CAD build for the part. Positions are in the model's coordinates, mm. A direction names the side the tool comes from. Coordinates: 2 decimals unless noted, no trailing zeros. Loops run counter-clockwise (first coordinate to the right, second up) from the corner with the lowest first, then second, coordinate; pieces in that order, holes last. Notation, with made-up numbers: (8, -19) -> (31, -19) arc R27 ccw to (31, 14) -> close; hole circle Ø4 at (-24.5, 32.25). An arc over 180 degrees is marked (long way). Write each question's results on one line, items separated by ' | '.
from build123d import *

# Parameters (mm, degrees)
SKETCH1_R               = 42.75
SKETCH1_R_2             = 38.75
BOSS_EXTRUDE1_DEPTH     = 20
BOSS_EXTRUDE2_DEPTH     = 15
SKETCH3_R               = 1.75
CUT_EXTRUDE1_DEPTH      = 43.75
CUT_EXTRUDE1_DEPTH_BACK = 43.75
SKETCH4_R               = 1.75
CUT_EXTRUDE2_DEPTH      = 43.7500001
CUT_EXTRUDE2_DEPTH_BACK = 43.7500001
FILLET1_R               = 2


with BuildPart() as part:
    # Sketch1 → Boss-Extrude1 (new body)
    with BuildSketch(Plane(origin=(0, 0, 0), x_dir=(1, 0, 0), z_dir=(0, 1, 0))):
        Circle(SKETCH1_R)
        Circle(SKETCH1_R_2, mode=Mode.SUBTRACT)
    extrude(amount=BOSS_EXTRUDE1_DEPTH)

    # Sketch2 → Boss-Extrude2 (add)
    with BuildSketch(Plane.XZ):
        with BuildLine():
            Line((40.171859539, 14.621361127), (36.413089055, 13.253280554))
            ThreePointArc((36.413089055, 13.253280554), (38.161300429, 6.728866885), (38.75, 0))
            Line((38.75, 0), (42.75, 0))
            ThreePointArc((42.75, 0), (42.100531441, 7.423459595), (40.171859539, 14.621361127))
        make_face()
        with BuildLine():
            Line((-7.423459595, -42.100531441), (-6.728866885, -38.161300429))
            ThreePointArc((-6.728866885, -38.161300429), (-13.253280554, -36.413089056), (-19.375, -33.558484397))
            Line((-19.375, -33.558484397), (-21.375, -37.022586012))
            ThreePointArc((-21.375, -37.022586012), (-14.621361127, -40.171859539), (-7.423459595, -42.100531441))
        make_face()
        with BuildLine():
            Line((-32.748399943, 27.479170314), (-29.684222171, 24.908019875))
            ThreePointArc((-29.684222171, 24.908019875), (-24.908019875, 29.684222171), (-19.375, 33.558484397))
            Line((-19.375, 33.558484397), (-21.375, 37.022586012))
            ThreePointArc((-21.375, 37.022586012), (-27.479170314, 32.748399943), (-32.748399943, 27.479170314))
        make_face()
    extrude(amount=BOSS_EXTRUDE2_DEPTH)

    # Sketch3 → Cut-Extrude1 (cut, two sides)
    with BuildSketch(Plane.XY) as cut_extrude1_sk:
        with Locations((0, 10)):
            Circle(SKETCH3_R)
    extrude(amount=CUT_EXTRUDE1_DEPTH, mode=Mode.SUBTRACT)
    extrude(cut_extrude1_sk.sketch, amount=-CUT_EXTRUDE1_DEPTH_BACK, mode=Mode.SUBTRACT)

    # Sketch4 → Cut-Extrude2 (cut, two sides)
    with BuildSketch(Plane(origin=(0, 0, 0), x_dir=(0, 0, -1), z_dir=(1, 0, 0))) as cut_extrude2_sk:
        with Locations((0, 10)):
            Circle(SKETCH4_R)
    extrude(amount=CUT_EXTRUDE2_DEPTH, mode=Mode.SUBTRACT)
    extrude(cut_extrude2_sk.sketch, amount=-CUT_EXTRUDE2_DEPTH_BACK, mode=Mode.SUBTRACT)

    # Fillet1
    fillet1_edges = [part.edges().sort_by_distance(p)[0] for p in [
        (-42.75, 20, 0),
    ]]
    fillet(fillet1_edges, radius=FILLET1_R)


solid = part.part
1) Slice it at C-C (y = 10). Write the cut outline in (x, z), then the cut area to 3 significant figures.
Outcome:
outline: (-42.71, -1.75) arc R42.75 ccw to (-1.75, -42.71) -> (-1.75, -38.71) arc R38.75 cw to (-38.71, -1.75) -> close; (-42.71, 1.75) -> (-38.71, 1.75) arc R38.75 cw to (-1.75, 38.71) -> (-1.75, 42.71) arc R42.75 ccw to start; (1.75, -42.71) arc R42.75 ccw to (42.71, -1.75) -> (38.71, -1.75) arc R38.75 cw to (1.75, -38.71) -> close; (1.75, 38.71) arc R38.75 cw to (38.71, 1.75) -> (42.71, 1.75) arc R42.75 ccw to (1.75, 42.71) -> close | area: 968 mm^2
2) Pin check, flat tips, straight feed: pin 1 (21.5 mm diameter, centred on x = 21.5, z = -26, fed in from -Y); pin 2 (1.2 mm diameter, centred on x = 40, y = -9, fed in from -Z); pin 3 (8 mm diameter, centred on y = 13, z = -32.5, fed in from +X); pin 4 (3 mm diameter, centred on y = 10, z = 0, fed in from -X). Stop position of each tip, or through.
Outcome:
pin 1: stops at y = 0 | pin 2: stops at z = 0 | pin 3: stops at x = 31.86 | pin 4: passes through
3) Drill centre lines: L1, parallel to X at y = 12, z = 0; L2, parallel to Y at x = 0, z = 40.3; L3, parallel to Z at x = 30.5, y = 16. Where is each one in solid material? Low to high. Write a range as from..to.
Outcome:
L1: x = -42.75..-38.75, 38.75..42.75 | L2: y = 0..8.25, 11.75..20 | L3: z = -29.96..-23.9, 23.9..29.96
4) Slice it at A-A (x = 0). Write the cut outline in (y, z), then the cut area to 3 significant figures.
Outcome:
outline: (0, -42.75) -> (8.25, -42.75) -> (8.25, -38.75) -> (0, -38.75) -> close; (0, 38.75) -> (8.25, 38.75) -> (8.25, 42.75) -> (0, 42.75) -> close; (11.75, -42.75) -> (18, -42.75) arc R2 ccw to (20, -40.75) -> (20, -38.75) -> (11.75, -38.75) -> close; (11.75, 38.75) -> (20, 38.75) -> (20, 40.75) arc R2 ccw to (18, 42.75) -> (11.75, 42.75) -> close | area: 130 mm^2
5) Slice it at B-B (y = -2.5). Write the cut outline in (x, z) (3 decimals), then the cut area to 3 significant figures.
Outcome:
outline: (-32.748, 27.479) -> (-29.684, 24.908) arc R38.75 cw to (-19.375, 33.558) -> (-21.375, 37.023) arc R42.75 ccw to start; (-21.375, -37.023) arc R42.75 ccw to (-7.423, -42.101) -> (-6.729, -38.161) arc R38.75 cw to (-19.375, -33.558) -> close; (36.413, 13.253) arc R38.75 cw to (38.75, 0) -> (42.75, 0) arc R42.75 ccw to (40.172, 14.621) -> close | area: 171 mm^2
6) Two-plate mould, pull along X, no slides. Class faces 5 (the flat face through (-20.361, -7.395, 35.266)), 6 (the flat face through (25, 0, -31)), 7 (the flat face through (-20.361, -7.395, -35.266)), 8 (the cylindrical face through (-0.228, 11.735, -40.702)): pulls with the +X half, pulls with the -X half, needs draft (parallel to the pull), parting line crosses it, or undercut.
Outcome:
face 5: pulls with the +X half | face 6: needs draft | face 7: pulls with the -X half | face 8: undercut
7) Which spindle directions (+Z, -Z, +X, -X, +Y, -Y) get a long thin tool onto all of the face, cutting with end or side? Do faces 1 (the flat face through (38.319, -7.395, 13.947)), 2 (the flat face through (41, -7, 0)), 3 (the flat face through (-31.238, -7.395, 26.212)), 4 (the flat face through (-7.08, -7.4, -40.16)). Say none if no direction does.
Outcome:
face 1: +Z, -X, -Y | face 2: -Z, +X, -X, -Y | face 3: -Z, -X, -Y | face 4: -Z, +X, -Y
